Geometry check sheet. Reference: the model listing, model coordinates, mm. Face numbers are marked on the shaded views. Round coordinates to 2 decimals unless told otherwise and drop trailing zeros. Loops run counter-clockwise (first coordinate to the right, second up) from the corner with the lowest first, then second, coordinate; pieces in that order, holes last.
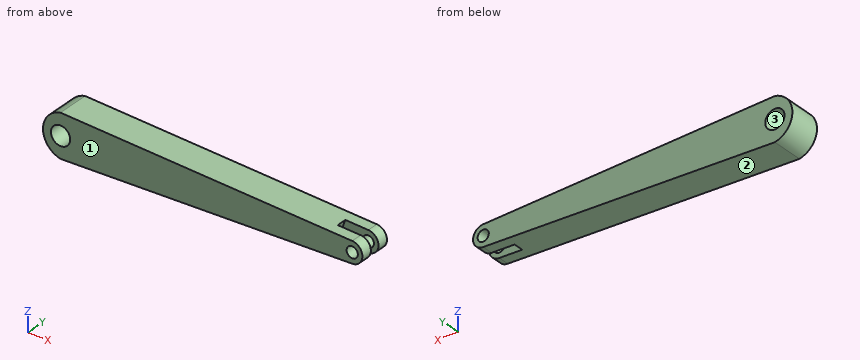
```python
from build123d import *

# Parameters (mm, degrees)
SKETCH1_R           = 1.75
SKETCH1_R_2         = 3
BOSS_EXTRUDE1_DEPTH = 10
SKETCH2_W           = 8
SKETCH2_H           = 3.1


with BuildPart() as part:
    # Sketch1 → Boss-Extrude1 (new body)
    with BuildSketch(Plane(origin=(0, 0, 0), x_dir=(1, 0, 0), z_dir=(0, 1, 0))):
        with BuildLine():
            Line((-24.049180328, 6.7), (66.950819672, 3.3))
            ThreePointArc((66.950819672, 3.3), (70.129825511, 0), (66.950819672, -3.3))
            Line((66.950819672, -3.3), (-24.049180328, -6.7))
            ThreePointArc((-24.049180328, -6.7), (-29.521356494, 0), (-24.049180328, 6.7))
        make_face()
        with Locations((66.950819672, 0)):
            Circle(SKETCH1_R, mode=Mode.SUBTRACT)
        with Locations((-24.049180328, 0)):
            Circle(SKETCH1_R_2, mode=Mode.SUBTRACT)
    extrude(amount=BOSS_EXTRUDE1_DEPTH)

    # Sketch2 → Cut-Revolve1 (revolve, cut)
    with BuildSketch(Plane(origin=(66.950819672, 0, 0), x_dir=(0, 0, -1), z_dir=(1, 0, 0))):
        with Locations((4, 5)):
            Rectangle(SKETCH2_W, SKETCH2_H)
    revolve(axis=Axis((66.950819672, 3.45, 0), (0, 1, 0)), mode=Mode.SUBTRACT)


solid = part.part
```
1) Scan lines: line 1 along X through (y, z) = (2.75, -0.5); line 2 along X through (y, z) = (8.5, -1.25); line 3 along Z through (x, y) = (36, 5.25). Record each from-to range of solid material in increasing order.
Report:
line 1: x = -29.5 to -27.01, -21.09 to 65.27, 68.63 to 70.09
line 2: x = -29.41 to -26.78, -21.32 to 65.73, 68.18 to 69.88
line 3: z = -4.46 to 4.46
2) Sectioned sample at B-B, the plane y = 7.5. Record the cut outline in (x, z).
Report:
outline: (-24.05, -6.7) - (66.95, -3.3) arc R3.3 ccw to (66.95, 3.3) - (-24.05, 6.7) arc R6.84 ccw to start; hole circle Ø6 at (-24.05, 0); hole circle Ø3.5 at (66.95, 0)
3) Gauge pin test, flat ends, axial feed: pin 1 (1 mm diameter, centred on y = 5, z = 0, fed in from +X); pin 2 (6 mm diameter, centred on y = 7, z = -3.5, fed in from +X); pin 3 (6 mm diameter, centred on x = 57.5, y = 2.5, fed in from -Z). Record the tip position at first contact, or that the pin passes through.
Report:
pin 1: stops at x = 58.97
pin 2: stops at x = 70.09
pin 3: stops at z = -3.77
4) Mould release check, pull along X, two halves, no side actions. Record for the marked faces 1, 2 and 3: +X half, -X half, draft (parallel to the pull), parting line (faces both ways), or undercut.
Report:
face 1: draft
face 2: +X half
face 3: undercut
5) Sectioned sample at C-C, the plane x = 7. Record the cut outline in (y, z), then the cut area to 3 significant figures.
Report:
outline: (0, -5.54) - (10, -5.54) - (10, 5.54) - (0, 5.54) - close
area: 111 mm2
6) Sectioned sample at D-D, the plane z = -4.5. Record the cut outline in (x, y), then the cut area to 3 significant figures.
Report:
outline: (-27.83, 0) - (34.83, 0) - (34.83, 10) - (-27.83, 10) - close
area: 627 mm2
7) Sectioned sample at A-A, the plane z = 0. Record the cut outline in (x, y), then the cut area to 3 significant figures.
Report:
outline: (-29.52, 0) - (-27.05, 0) - (-27.05, 10) - (-29.52, 10) - close; (-21.05, 0) - (65.2, 0) - (65.2, 3.45) - (58.95, 3.45) - (58.95, 6.55) - (65.2, 6.55) - (65.2, 10) - (-21.05, 10) - close; (68.7, 0) - (70.13, 0) - (70.13, 3.45) - (68.7, 3.45) - close; (68.7, 6.55) - (70.13, 6.55) - (70.13, 10) - (68.7, 10) - close
area: 878 mm2
